For this review, take the finished solid that the model builds, in its own axes (mm). A direction names the side the tool comes from. Round coordinates to 2 decimals unless told otherwise and drop trailing zeros. Loops run counter-clockwise (first coordinate to the right, second up) from the corner with the lowest first, then second, coordinate; pieces in that order, holes last. Notation, with made-up numbers: (52, 45.5) -> (107, 45.5) arc R11 cw to (107, 60.5) -> close; hole circle Ø11 at (87.5, 84). An arc over 180 degrees is marked (long way). One line per question, with ' | ' between items. Start each with the question number.
1. For pin 1 Ø1 at (y, z) = (88.5, 16.5) entering from -X; pin 2 Ø2 at (x, z) = (148.5, 23.5) entering from +Y; pin 3 Ø3.5 at (x, y) = (150.77, 87.35) entering from -Z; pin 4 Ø2 at (x, z) = (144.5, 6.5) entering from +Y, all flat-tipped, find the tip position at first contact; note any pin that passes through.
2. For faces 1 (the face through (155.2, 91.4, 36.4)), 2 (the face through (151, 85, 0)), list the 3-axis set-ups (+Z, -Z, +X, -X, +Y, -Y) from which the entire face can be reached by the end or side of a thin tool; tool diameter is ignored.
3. Wall thickness on line 1 along X through (y, z) = (87.5, 50); line 2 along X through (y, z) = (86.75, 58.5); line 3 along Y through (x, z) = (149.5, 28.5): over which ranges is each line inside the solid? List them lowest first.
4. Consider section A-A (z = 60). Write out the cut boundary in (x, y), and give its area (3 significant figures).
```python
from build123d import *

# Parameters (mm, degrees)
SKETCH_1_R      = 8.966016308
SKETCH_1_R_2    = 1.4
EXTRUDE_1_DEPTH = 3
SKETCH_2_R      = 6
SKETCH_2_R_2    = 1.4
EXTRUDE_2_DEPTH = 66
FILLET_1_R      = 5


with BuildPart() as part:
    # Эскиз1 → Бобышка-Вытянуть1 (new body)
    with BuildSketch(Plane.XY):
        with Locations((150.771693647, 87.352480595)):
            Circle(SKETCH_1_R)
        with Locations((150.771693647, 87.352480595)):
            Circle(SKETCH_1_R_2, mode=Mode.SUBTRACT)
    extrude(amount=EXTRUDE_1_DEPTH)

    # Эскиз2 → Бобышка-Вытянуть2 (add)
    with BuildSketch(Plane(origin=(0, 0, 0), x_dir=(-1, 0, 0), z_dir=(0, 0, -1))):
        with Locations((-150.771693647, 87.352480595)):
            Circle(SKETCH_2_R)
        with Locations((-150.771693647, 87.352480595)):
            Circle(SKETCH_2_R_2, mode=Mode.SUBTRACT)
    extrude(amount=-EXTRUDE_2_DEPTH)

    # Скругление1
    # the kernel refuses this fillet: 5 mm, written as the material it adds along each edge
    with BuildSketch(Plane(origin=(150.771693647, 87.352480595, 3), x_dir=(-1, 0, 0), z_dir=(0, -1, 0))) as fillet_1_piece_1:
        with BuildLine():
            CenterArc((11, -4.567593495), FILLET_1_R, 114.00376912, 65.99623088)
            Line((6, -4.567593495), (5.9, -4.567593495))
            Line((5.9, -4.567593495), (5.9, 0))
            Line((5.9, 0), (6, 0.1))
            ThreePointArc((6, 0.1), (7.483008154, 0.1), (8.925336634, 0.09135187))
            Line((8.925336634, 0.09135187), (8.966016308, 0))
        make_face()
    revolve(axis=Axis((150.771693647, 87.352480595, 3), (0, 0, -1)))


solid = part.part
```
Answer block:
1) pin 1: stops at x = 144.81 | pin 2: stops at y = 93.22 | pin 3: stops at z = 0 | pin 4: stops at y = 90.52
2) face 1: +Z | face 2: -Z, +X, -X, +Y, -Y
3) line 1: x = 144.77 to 149.38, 152.16 to 156.77 | line 2: x = 144.8 to 149.51, 152.04 to 156.74 | line 3: y = 81.49 to 86.77, 87.94 to 93.22
4) outline: circle Ø12 at (150.77, 87.35); hole circle Ø2.8 at (150.77, 87.35) | area: 107 mm2
